from build123d import *

# Parameters (mm, degrees)
CYLINDER135_R             = 1.7
CYLINDER135_DEPTH         = 16
CYLINDER136_R             = 1.7
CYLINDER136_DEPTH         = 16
CYLINDER137_R             = 1.7
CYLINDER137_DEPTH         = 16
CYLINDER138_R             = 1.7
CYLINDER138_DEPTH         = 16
CYLINDER083_R             = 3.5
CYLINDER083_DEPTH         = 2.5
BOX028_W                  = 29.5
BOX028_H                  = 2.5
BOX028_DEPTH              = 12
CYLINDER085_R             = 3.5
CYLINDER085_DEPTH         = 2.5
BOX034_W                  = 29.5
BOX034_H                  = 2.5
BOX034_DEPTH              = 12
CYLINDER086_R             = 3.5
CYLINDER086_DEPTH         = 2.5
BOX018_W                  = 2.5
BOX018_H                  = 21
BOX018_DEPTH              = 12
BOX042_W                  = 4
BOX042_H                  = 4
BOX042_DEPTH              = 12
FILLET002_R               = 2
FILLET002_PLACEMENT_ANGLE = 90
BOX040_W                  = 4
BOX040_H                  = 4
BOX040_DEPTH              = 12
FILLET_R                  = 2
BOX041_W                  = 4
BOX041_H                  = 4
BOX041_DEPTH              = 12
FILLET001_R               = 2
FILLET001_PLACEMENT_ANGLE = 90
BOX043_W                  = 4
BOX043_H                  = 4
BOX043_DEPTH              = 12
FILLET003_R               = 2
FILLET003_PLACEMENT_ANGLE = 180
CYLINDER129_R             = 3.5
CYLINDER129_DEPTH         = 2.5
BOX070_W                  = 2.5
BOX070_H                  = 21
BOX070_DEPTH              = 12
FILLET008_R               = 2


with BuildPart() as cylinder135:
    # Cylinder135 → Cylinder135 (new body)
    with BuildSketch(Plane(origin=(-10, -10.5, 0), x_dir=(1, 0, 0), z_dir=(0, 0, 1))):
        Circle(CYLINDER135_R)
    extrude(amount=CYLINDER135_DEPTH)


with BuildPart() as cylinder136:
    # Cylinder136 → Cylinder136 (new body)
    with BuildSketch(Plane(origin=(-10, -29.5, 0), x_dir=(1, 0, 0), z_dir=(0, 0, 1))):
        Circle(CYLINDER136_R)
    extrude(amount=CYLINDER136_DEPTH)


with BuildPart() as cylinder137:
    # Cylinder137 → Cylinder137 (new body)
    with BuildSketch(Plane(origin=(12.5, -10.5, 0), x_dir=(1, 0, 0), z_dir=(0, 0, 1))):
        Circle(CYLINDER137_R)
    extrude(amount=CYLINDER137_DEPTH)


with BuildPart() as fusion099:
    # Cylinder138 → Cylinder138 (new body)
    with BuildSketch(Plane(origin=(12.5, -29.5, 0), x_dir=(1, 0, 0), z_dir=(0, 0, 1))):
        Circle(CYLINDER138_R)
    extrude(amount=CYLINDER138_DEPTH)

    # Fusion099: union Cylinder135, Cylinder136, Cylinder137
    add(cylinder135.part)
    add(cylinder136.part)
    add(cylinder137.part)


with BuildPart() as cylinder083:
    # Cylinder083 → Cylinder083 (new body)
    with BuildSketch(Plane.XZ.offset(55.5)):
        Circle(CYLINDER083_R)
    extrude(amount=CYLINDER083_DEPTH)


with BuildPart() as cut037:
    # Box028 → Box028 (new body)
    with BuildSketch(Plane(origin=(-13.5, -58, 0), x_dir=(1, 0, 0), z_dir=(0, 0, 1))):
        with Locations((14.75, 1.25)):
            Rectangle(BOX028_W, BOX028_H)
    extrude(amount=BOX028_DEPTH)

    # Cut037: cut Cylinder083
    add(cylinder083.part, mode=Mode.SUBTRACT)


with BuildPart() as cut037_1:
    # Cut037 placement: moved
    add(cut037.part.moved(Location((0, 25, 0))))


with BuildPart() as cylinder085:
    # Cylinder085 → Cylinder085 (new body)
    with BuildSketch(Plane.XZ.offset(55.5)):
        Circle(CYLINDER085_R)
    extrude(amount=CYLINDER085_DEPTH)


with BuildPart() as cut039:
    # Box034 → Box034 (new body)
    with BuildSketch(Plane(origin=(-13.5, -58, 0), x_dir=(1, 0, 0), z_dir=(0, 0, 1))):
        with Locations((14.75, 1.25)):
            Rectangle(BOX034_W, BOX034_H)
    extrude(amount=BOX034_DEPTH)

    # Cut039: cut Cylinder085
    add(cylinder085.part, mode=Mode.SUBTRACT)


with BuildPart() as cut039_1:
    # Cut039 placement: moved
    add(cut039.part.moved(Location((0, 48.5, 0))))


with BuildPart() as cylinder086:
    # Cylinder086 → Cylinder086 (new body)
    with BuildSketch(Plane(origin=(-11, -20, 12), x_dir=(0, 0, 1), z_dir=(-1, 0, 0))):
        Circle(CYLINDER086_R)
    extrude(amount=CYLINDER086_DEPTH)


with BuildPart() as cut075:
    # Box018 → Box018 (new body)
    with BuildSketch(Plane(origin=(-13.5, -30.5, 0), x_dir=(1, 0, 0), z_dir=(0, 0, 1))):
        with Locations((1.25, 10.5)):
            Rectangle(BOX018_W, BOX018_H)
    extrude(amount=BOX018_DEPTH)

    # Cut075: cut Cylinder086
    add(cylinder086.part, mode=Mode.SUBTRACT)


with BuildPart() as cut075_1:
    # Cut075 placement: moved
    add(cut075.part.moved(Location((27, 0, 0))))


with BuildPart() as fillet002:
    # Box042 → Box042 (new body)
    with BuildSketch(Plane(origin=(-11, -39, 0), x_dir=(1, 0, 0), z_dir=(0, 0, 1))):
        with Locations((2, 2)):
            Rectangle(BOX042_W, BOX042_H)
    extrude(amount=BOX042_DEPTH)

    # Fillet002
    fillet002_edges = [fillet002.edges().sort_by_distance(p)[0] for p in [
        (-7, -39, 6),
    ]]
    fillet(fillet002_edges, radius=FILLET002_R)


with BuildPart() as fillet002_1:
    # Fillet002 placement: moved
    add(fillet002.part.moved(Location((48.5, -20.5, 0))).rotate(Axis((48.5, -20.5, 0), (0, 0, -1)), FILLET002_PLACEMENT_ANGLE))


with BuildPart() as fillet_body:
    # Box040 → Box040 (new body)
    with BuildSketch(Plane(origin=(-11, -39, 0), x_dir=(1, 0, 0), z_dir=(0, 0, 1))):
        with Locations((2, 2)):
            Rectangle(BOX040_W, BOX040_H)
    extrude(amount=BOX040_DEPTH)

    # Fillet
    fillet_edges = [fillet_body.edges().sort_by_distance(p)[0] for p in [
        (-7, -39, 6),
    ]]
    fillet(fillet_edges, radius=FILLET_R)


with BuildPart() as fillet_body_1:
    # Fillet placement: moved
    add(fillet_body.part.moved(Location((0, 25.5, 0))))


with BuildPart() as fillet001:
    # Box041 → Box041 (new body)
    with BuildSketch(Plane(origin=(-11, -39, 0), x_dir=(1, 0, 0), z_dir=(0, 0, 1))):
        with Locations((2, 2)):
            Rectangle(BOX041_W, BOX041_H)
    extrude(amount=BOX041_DEPTH)

    # Fillet001
    fillet001_edges = [fillet001.edges().sort_by_distance(p)[0] for p in [
        (-7, -39, 6),
    ]]
    fillet(fillet001_edges, radius=FILLET001_R)


with BuildPart() as fillet001_1:
    # Fillet001 placement: moved
    add(fillet001.part.moved(Location((-46, -19.5, 0))).rotate(Axis((-46, -19.5, 0), (0, 0, 1)), FILLET001_PLACEMENT_ANGLE))


with BuildPart() as fillet003:
    # Box043 → Box043 (new body)
    with BuildSketch(Plane(origin=(-11, -39, 0), x_dir=(1, 0, 0), z_dir=(0, 0, 1))):
        with Locations((2, 2)):
            Rectangle(BOX043_W, BOX043_H)
    extrude(amount=BOX043_DEPTH)

    # Fillet003
    fillet003_edges = [fillet003.edges().sort_by_distance(p)[0] for p in [
        (-7, -39, 6),
    ]]
    fillet(fillet003_edges, radius=FILLET003_R)


with BuildPart() as fillet003_1:
    # Fillet003 placement: moved
    add(fillet003.part.moved(Location((2.5, -65.5, 0))).rotate(Axis((2.5, -65.5, 0), (0, 0, 1)), FILLET003_PLACEMENT_ANGLE))


with BuildPart() as cylinder129:
    # Cylinder129 → Cylinder129 (new body)
    with BuildSketch(Plane(origin=(-11, -20, 12), x_dir=(0, 0, 1), z_dir=(-1, 0, 0))):
        Circle(CYLINDER129_R)
    extrude(amount=CYLINDER129_DEPTH)


with BuildPart() as fillet008:
    # Box070 → Box070 (new body)
    with BuildSketch(Plane(origin=(-13.5, -30.5, 0), x_dir=(1, 0, 0), z_dir=(0, 0, 1))):
        with Locations((1.25, 10.5)):
            Rectangle(BOX070_W, BOX070_H)
    extrude(amount=BOX070_DEPTH)

    # Cut077: cut Cylinder129
    add(cylinder129.part, mode=Mode.SUBTRACT)

    # Fusion106: union Cut037, Cut039, Cut075, Fillet002, Fillet body, Fillet001, Fillet003
    add(cut037_1.part)
    add(cut039_1.part)
    add(cut075_1.part)
    add(fillet002_1.part)
    add(fillet_body_1.part)
    add(fillet001_1.part)
    add(fillet003_1.part)

    # Cut084: cut Fusion099
    add(fusion099.part, mode=Mode.SUBTRACT)

    # Fillet008
    fillet008_edges = [fillet008.edges().sort_by_distance(p)[0] for p in [
        (-13.5, -7, 6),
        (-13.5, -33, 6),
        (16, -7, 6),
        (16, -33, 6),
    ]]
    fillet(fillet008_edges, radius=FILLET008_R)


solid = fillet008.part
The listing builds one solid part. Answer for the finished solid, in the listing's coordinates (mm). A direction names the side the tool comes from. Give positions to 0.01 mm unless a question says otherwise; leave off trailing zeros. Loops run counter-clockwise (first coordinate to the right, second up) from the corner with the lowest first, then second, coordinate; pieces in that order, holes last. Notation, with made-up numbers: (-0.75, -7) - (8.25, -7) arc R21 cw to (8.25, 17) - close; hole circle Ø11 at (-24.5, 20). An arc over 180 degrees is marked (long way). Write each question's results on one line, items separated by ' | '.
1. Find section C-C, the plane x = 12.5. Write down the section's boundary in (y, z).
Resolved:
outline: (-33, 0) - (-31.2, 0) - (-31.2, 12) - (-33, 12) - close; (-27.8, 0) - (-26.5, 0) - (-26.5, 12) - (-27.8, 12) - close; (-13.5, 0) - (-12.2, 0) - (-12.2, 12) - (-13.5, 12) - close; (-8.8, 0) - (-7, 0) - (-7, 12) - (-8.8, 12) - close
2. For a pull along X with two mould halves and no side action, classify faces 3 (the face through (1, -7, 6)), 4 (the face through (10.07, -12.9, 6.08)), 5 (the face through (-13.5, -20, 6)) as +X half, -X half, draft (parallel to the pull), parting line (faces both ways), or undercut.
Resolved:
face 3: draft | face 4: undercut | face 5: -X half
3. Find section A-A, the plane y = -20. Write down the section's boundary in (x, z).
Resolved:
outline: (-13.5, 0) - (-11, 0) - (-11, 8.5) - (-13.5, 8.5) - close; (13.5, 0) - (16, 0) - (16, 8.5) - (13.5, 8.5) - close
4. Which of the six approach directions +Z, -Z, +X, -X, +Y, -Y give full straight-line access (tool end or side, diameter ignored) to faces 1 (the face through (0.1, -8.2, 3.5)), 2 (the face through (12, -13.5, 6))?
Resolved:
face 1: -Z, +Y, -Y | face 2: +Z, -Z
5. Find section B-B, the plane y = -29.5. Write down the section's boundary in (x, z), then the cut area to 3 significant figures.
Resolved:
outline: (-13.5, 0) - (-11.7, 0) - (-11.7, 12) - (-13.5, 12) - close; (-8.3, 0) - (-7, 0) - (-7, 12) - (-8.3, 12) - close; (9.5, 0) - (10.8, 0) - (10.8, 12) - (9.5, 12) - close; (14.2, 0) - (16, 0) - (16, 12) - (14.2, 12) - close | area: 74.4 mm^2
6. Consider probe 1 along Y at (x, z) = (12.5, 5); probe 2 along X at (y, z) = (-10.5, 3); probe 3 along X at (y, z) = (-20.5, 5). Determine where each line is inside the solid, lowest interval first. Write a range as from..to.
Resolved:
probe 1: y = -33..-31.2, -27.8..-26.5, -13.5..-12.2, -8.8..-7 | probe 2: x = -13.5..-11.7, -8.3..-7, 9.5..10.8, 14.2..16 | probe 3: x = -13.5..-11, 13.5..16
7. Find section D-D, the plane z = 5. Write down the section's boundary in (x, y).
Resolved:
outline: (-13.5, -31) arc R2 ccw to (-11.5, -33) - (14, -33) arc R2 ccw to (16, -31) - (16, -9) arc R2 ccw to (14, -7) - (-11.5, -7) arc R2 ccw to (-13.5, -9) - close; hole circle Ø3.4 at (-10, -29.5); hole circle Ø3.4 at (-10, -10.5); hole (-11, -26.5) - (-9, -26.5) arc R2 cw to (-7, -28.5) - (-7, -30.5) - (9.5, -30.5) - (9.5, -28.5) arc R2 cw to (11.5, -26.5) - (13.5, -26.5) - (13.5, -13.5) - (11.5, -13.5) arc R2 cw to (9.5, -11.5) - (9.5, -9.5) - (-7, -9.5) - (-7, -11.5) arc R2 cw to (-9, -13.5) - (-11, -13.5) - close; hole circle Ø3.4 at (12.5, -29.5); hole circle Ø3.4 at (12.5, -10.5)
